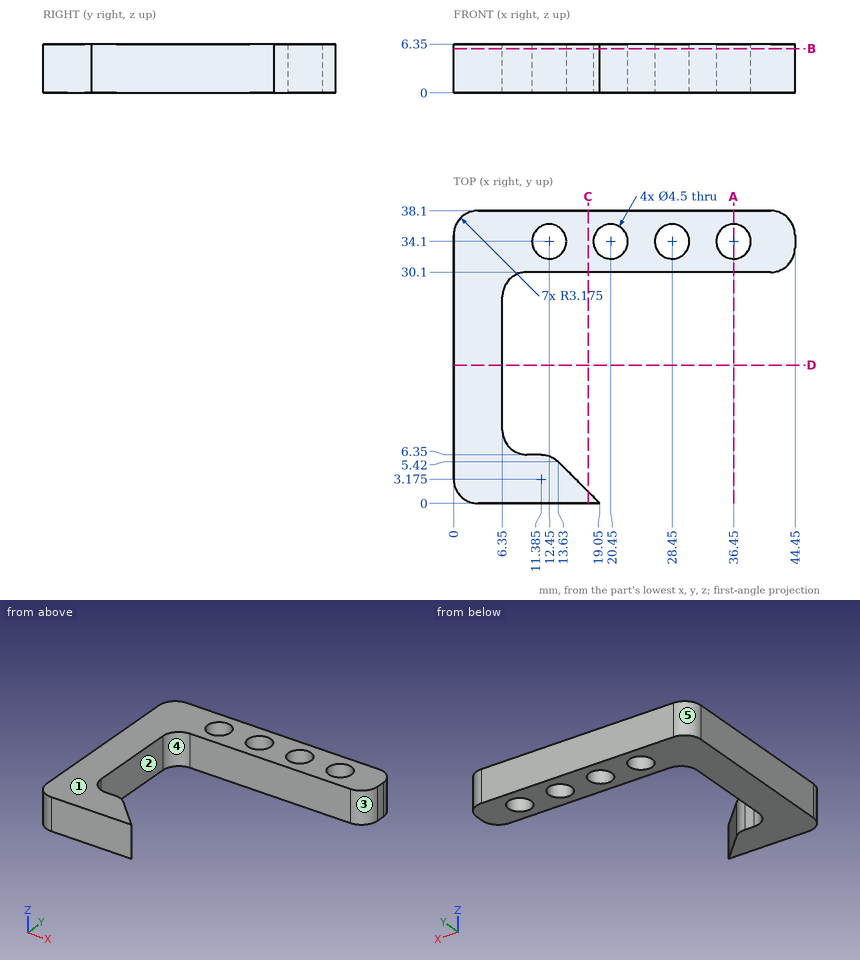
Geometry check sheet. Reference: drawing and pictorial views, mm from the part's lowest x, y, z. A direction names the side the tool comes from. Round coordinates to 2 decimals unless told otherwise and drop trailing zeros. Order: outer loops, then holes, each group sorted by start corner. A loop starts at its lowest first (then second) coordinate and runs counter-clockwise, first axis right, second up.
Q1. Scan lines: L1, parallel to Y at x = 36.45, z = 4.75; L2, parallel to X at y = 15, z = 1.5; L3, parallel to Y at x = 3, z = 6 (3 decimals). Record each from-to range of solid material in increasing order.
Filled sheet:
L1: y = 30.1 to 31.85, 36.35 to 38.1
L2: x = 0 to 6.35
L3: y = 0.005 to 38.095
Q2. Cross-section at B-B, the plane z = 5.75. Enter the section's corners in (x, y) (3 decimals).
Filled sheet:
outline: (0, 3.175) arc R3.175 ccw to (3.175, 0) - (19.05, 0) - (13.63, 5.42) arc R3.175 ccw to (11.385, 6.35) - (9.525, 6.35) arc R3.175 cw to (6.35, 9.525) - (6.35, 26.925) arc R3.175 cw to (9.525, 30.1) - (41.275, 30.1) arc R3.175 ccw to (44.45, 33.275) - (44.45, 34.925) arc R3.175 ccw to (41.275, 38.1) - (3.175, 38.1) arc R3.175 ccw to (0, 34.925) - close; hole circle Ø4.5 at (12.45, 34.1); hole circle Ø4.5 at (20.45, 34.1); hole circle Ø4.5 at (28.45, 34.1); hole circle Ø4.5 at (36.45, 34.1)
Q3. Depth check by flat-ended pin: P1, Ø6, axis at x = 12.45, y = 34.1, coming from the -Z side; P2, Ø3, axis at x = 22.5, z = 2, coming from the -Y side. Enter the tip coordinate at first touch or a pass-through.
Filled sheet:
P1: stops at z = 0
P2: stops at y = 30.1
Q4. Draft check along Y on the marked faces 1, 2 and 3. Enter one of: pulls with the +Y half, pulls with the -Y half, needs draft (parallel to the pull), parting line crosses it, or undercut.
Filled sheet:
face 1: needs draft
face 2: undercut
face 3: pulls with the -Y half
Q5. Cross-section at D-D, the plane y = 18. Enter the section's corners in (x, z).
Filled sheet:
outline: (0, 0) - (6.35, 0) - (6.35, 6.35) - (0, 6.35) - close
Q6. Cross-section at A-A, the plane x = 36.45. Enter the section's corners in (y, z), plus the area to 3 significant figures.
Filled sheet:
outline: (30.1, 0) - (31.85, 0) - (31.85, 6.35) - (30.1, 6.35) - close; (36.35, 0) - (38.1, 0) - (38.1, 6.35) - (36.35, 6.35) - close
area: 22.2 mm2
Q7. Set-up check for the marked faces 4 and 5: record each of +Z, -Z, +X, -X, +Y, -Y from which the full face is reachable in a straight line by a thin tool's end or side.
Filled sheet:
face 4: +Z, -Z, +X
face 5: +Z, -Z, -X, +Y
Q8. Cross-section at C-C, the plane x = 17.5. Enter the section's corners in (y, z).
Filled sheet:
outline: (0, 0) - (1.55, 0) - (1.55, 6.35) - (0, 6.35) - close; (30.1, 0) - (38.1, 0) - (38.1, 6.35) - (30.1, 6.35) - close
